Could you check a few things on this model? Use its own coordinates, in mm. Give positions to 0.01 mm unless a question says otherwise; leave off trailing zeros. Loops run counter-clockwise (first coordinate to the right, second up) from the corner with the lowest first, then second, coordinate; pieces in that order, holes last. Notation, with made-up numbers: (-32.75, 74.25) - (2.25, 74.25) arc R31 cw to (2.25, 112.25) - close; hole circle Ø8 at (53.25, 23.5). An arc over 180 degrees is marked (long way). One line per item, written item: value. Start each with the question number.
Q1. I want a section at A-A (x = -31.75). Please give me the cut outline in (y, z).
Q2. I want a section at D-D (z = 8.25). Please give me the cut outline in (x, y), then the cut area to 3 significant figures.
Q3. I'm going to push flat-ended pins straight in: P1, Ø5, axis at y = 1.5, z = 18, coming from the +X side; P2, Ø2, axis at y = 2.5, z = 16, coming from the +X side; P3, Ø4, axis at y = 3, z = 15.5, coming from the -X side; P4, Ø4, axis at x = -30.07, z = 13.37, coming from the -Y side. Where does each tip first touch, or does it pass through?
Q4. I want a section at C-C (y = 6.75). Please give me the cut outline in (x, z), then the cut area to 3 significant figures.
Q5. If I drill on line 1 (X direction, y = 2.25, z = 13.5); line 2 (Z direction, x = -29.75, y = 3); line 3 (X direction, y = 5.5, z = 13.75), over which ranges is the centre line in solid material (lowest first)? Write a range as from..to.
Q6. I want a section at B-B (z = 15). Please give me the cut outline in (x, y).
```python
from build123d import *

# Parameters (mm, degrees)
F1_DEPTH = 8
F2_DEPTH = 3
F3_DEPTH = 11


with BuildPart() as f1:
    # F0 (on Front) → F1 (new body)
    with BuildSketch(Plane.XZ):
        with BuildLine():
            ThreePointArc((-30.070162, 46.37237), (-35.632137, 46.568408), (-41.166509, 47.155549))
            ThreePointArc((-41.166509, 47.155549), (-30.070162, -22.199768), (-18.973814, 47.155549))
            ThreePointArc((-18.973814, 47.155549), (-24.508186, 46.568408), (-30.070162, 46.37237))
        make_face()
        with BuildLine():
            ThreePointArc((-22.570162, 13.365558), (-35.373463, 8.062257), (-30.070162, 20.865558))
            ThreePointArc((-30.070162, 20.865558), (-24.766861, 18.668859), (-22.570162, 13.365558))
        make_face(mode=Mode.SUBTRACT)
    extrude(amount=F1_DEPTH)

    # F0 (on Front) → F2 (join)
    with BuildSketch(Plane.XZ):
        with BuildLine():
            ThreePointArc((-30.070162, 56.279502), (-36.966771, 53.357463), (-41.166509, 47.155549))
            ThreePointArc((-41.166509, 47.155549), (-35.632137, 46.568408), (-30.070162, 46.37237))
            Line((-30.070162, 46.37237), (-30.070162, 50.721558))
            ThreePointArc((-30.070162, 50.721558), (-32.070162, 52.721558), (-30.070162, 54.721558))
            Line((-30.070162, 54.721558), (-30.070162, 56.279502))
        make_face()
        with BuildLine():
            ThreePointArc((-30.070162, 46.37237), (-24.508186, 46.568408), (-18.973814, 47.155549))
            ThreePointArc((-18.973814, 47.155549), (-23.173552, 53.357463), (-30.070162, 56.279502))
            Line((-30.070162, 56.279502), (-30.070162, 54.721558))
            ThreePointArc((-30.070162, 54.721558), (-28.655948, 54.135772), (-28.070162, 52.721558))
            ThreePointArc((-28.070162, 52.721558), (-28.655948, 51.307344), (-30.070162, 50.721558))
            Line((-30.070162, 50.721558), (-30.070162, 46.37237))
        make_face()
    extrude(amount=F2_DEPTH)


with BuildPart() as f3:
    # F0 (on Front) → F3 (new body)
    with BuildSketch(Plane.XZ):
        with BuildLine():
            ThreePointArc((-22.570162, 13.365558), (-24.766861, 18.668859), (-30.070162, 20.865558))
            ThreePointArc((-30.070162, 20.865558), (-35.373463, 8.062257), (-22.570162, 13.365558))
        make_face()
        with BuildLine():
            ThreePointArc((-27.570162, 13.365558), (-31.837929, 11.597791), (-30.070162, 15.865558))
            ThreePointArc((-30.070162, 15.865558), (-28.302395, 15.133325), (-27.570162, 13.365558))
        make_face(mode=Mode.SUBTRACT)
    extrude(amount=-F3_DEPTH)


solid = f3.part
```
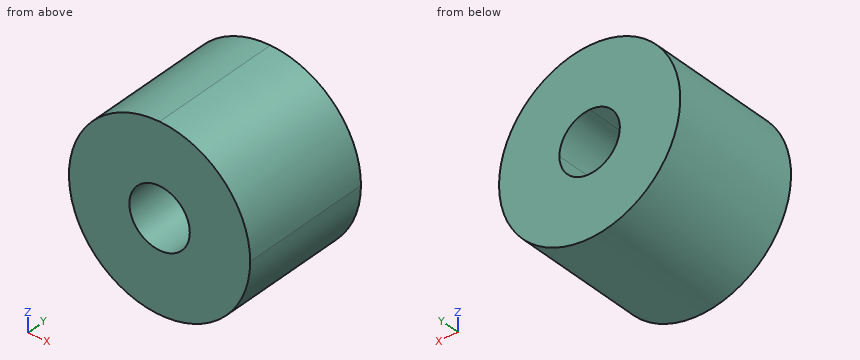
Worked answers:
1. outline: (0, 6.06) - (11, 6.06) - (11, 11.51) - (0, 11.51) - close; (0, 15.22) - (11, 15.22) - (11, 20.68) - (0, 20.68) - close
2. outline: (-35.55, 0) - (-24.59, 0) - (-24.59, 11) - (-35.55, 11) - close
2. area: 121 mm²
3. P1: stops at x = -22.88
3. P2: stops at x = -22.75
3. P3: stops at x = -37.57
3. P4: passes through
4. outline: circle Ø15 at (-30.07, 13.37); hole circle Ø5 at (-30.07, 13.37)
4. area: 157 mm²
5. line 1: x = -37.57..-32.57, -27.57..-22.57
5. line 2: z = 5.87..10.89, 15.84..20.86
5. line 3: x = -37.56..-32.54, -27.6..-22.58
6. outline: (-37.39, 0) - (-31.96, 0) - (-31.96, 11) - (-37.39, 11) - close; (-28.18, 0) - (-22.75, 0) - (-22.75, 11) - (-28.18, 11) - close
